```python
from build123d import *

# Parameters (mm, degrees)
F0_R     = 3.81
F1_DEPTH = 1.27


with BuildPart() as f1:
    # F0 (on Top) → F1 (new body)
    with BuildSketch(Plane.XY):
        with BuildLine():
            ThreePointArc((8.255, -3.299557), (8.729807, -1.680052), (8.89, 0))
            ThreePointArc((8.89, 0), (8.729807, 1.680052), (8.255, 3.299557))
            ThreePointArc((8.255, 3.299557), (7.698966, 4.445), (6.985, 5.499261))
            ThreePointArc((6.985, 5.499261), (4.445, 7.698966), (1.27, 8.798818))
            ThreePointArc((1.27, 8.798818), (0, 8.89), (-1.27, 8.798818))
            ThreePointArc((-1.27, 8.798818), (-4.445, 7.698966), (-6.985, 5.499261))
            ThreePointArc((-6.985, 5.499261), (-7.698966, 4.445), (-8.255, 3.299557))
            ThreePointArc((-8.255, 3.299557), (-8.89, 0), (-8.255, -3.299557))
            ThreePointArc((-8.255, -3.299557), (-7.698966, -4.445), (-6.985, -5.499261))
            ThreePointArc((-6.985, -5.499261), (-4.445, -7.698966), (-1.27, -8.798818))
            ThreePointArc((-1.27, -8.798818), (0, -8.89), (1.27, -8.798818))
            ThreePointArc((1.27, -8.798818), (4.445, -7.698966), (6.985, -5.499261))
            ThreePointArc((6.985, -5.499261), (7.698966, -4.445), (8.255, -3.299557))
        make_face()
        Circle(F0_R, mode=Mode.SUBTRACT)
        with BuildLine():
            ThreePointArc((-1.27, 8.798818), (0, 8.89), (1.27, 8.798818))
            Line((1.27, 8.798818), (1.27, 11.338818))
            Line((1.27, 11.338818), (-1.27, 11.338818))
            Line((-1.27, 11.338818), (-1.27, 8.798818))
        make_face()
        with BuildLine():
            ThreePointArc((6.985, 5.499261), (7.698966, 4.445), (8.255, 3.299557))
            Line((8.255, 3.299557), (10.454705, 4.569557))
            Line((10.454705, 4.569557), (9.184705, 6.769261))
            Line((9.184705, 6.769261), (6.985, 5.499261))
        make_face()
        with BuildLine():
            Line((10.454705, -4.569557), (8.255, -3.299557))
            ThreePointArc((8.255, -3.299557), (7.698966, -4.445), (6.985, -5.499261))
            Line((6.985, -5.499261), (9.184705, -6.769261))
            Line((9.184705, -6.769261), (10.454705, -4.569557))
        make_face()
        with BuildLine():
            Line((1.27, -11.338818), (1.27, -8.798818))
            ThreePointArc((1.27, -8.798818), (0, -8.89), (-1.27, -8.798818))
            Line((-1.27, -8.798818), (-1.27, -11.338818))
            Line((-1.27, -11.338818), (1.27, -11.338818))
        make_face()
        with BuildLine():
            Line((-9.184705, -6.769261), (-6.985, -5.499261))
            ThreePointArc((-6.985, -5.499261), (-7.698966, -4.445), (-8.255, -3.299557))
            Line((-8.255, -3.299557), (-10.454705, -4.569557))
            Line((-10.454705, -4.569557), (-9.184705, -6.769261))
        make_face()
        with BuildLine():
            ThreePointArc((-8.255, 3.299557), (-7.698966, 4.445), (-6.985, 5.499261))
            Line((-6.985, 5.499261), (-9.184705, 6.769261))
            Line((-9.184705, 6.769261), (-10.454705, 4.569557))
            Line((-10.454705, 4.569557), (-8.255, 3.299557))
        make_face()
    extrude(amount=F1_DEPTH)


solid = f1.part
```
The listing builds one solid part. Answer for the finished solid, in the listing's coordinates (mm). A direction names the side the tool comes from. Give positions to 0.01 mm unless a question says otherwise; leave off trailing zeros. Order: outer loops, then holes, each group sorted by start corner. A loop starts at its lowest first (then second) coordinate and runs counter-clockwise, first axis right, second up. Notation, with made-up numbers: (-23.75, 82) -> (-11.75, 82) arc R24 cw to (-11.75, 117) -> close; hole circle Ø8 at (31.25, 54). An arc over 180 degrees is marked (long way). Answer as a JSON object with one key per item and string values. Group by question number.
Item 1: The part is cut by section A-A on x = 0. Write down the section's boundary in (y, z).
Item 2: Consider L1, parallel to Y at x = 0, z = 0.6; L2, parallel to X at y = 6.5, z = 0.1; L3, parallel to X at y = -0.75, z = 0.5. Determine where each line is inside the solid, lowest interval first. Write a range as from..to.
Item 3: The part is cut by section D-D on y = 10.25. Write down the section's boundary in (x, z), and give its area (3 significant figures).
Item 4: Determine the mould class of faces 5 (the flat face through (9.37, -3.943, 0.626)), 6 (the flat face through (-9.8, 5.7, 0.6)), 7 (the flat face through (1.27, 10, 1)) for opening direction Y: pulls with the +Y half, pulls with the -Y half, needs draft (parallel to the pull), parting line crosses it, or undercut.
Item 5: A tool of negligible diameter and unlimited length cuts with its end or side. For faces 1 (the flat face through (1.27, -10, 1)), 2 (the cylindrical face through (-4.404, 7.723, 0.626)), 3 (the flat face through (-1.27, 10, 1)), 4 (the flat face through (-8.1, -6.143, 0.626)), from which of +Z, -Z, +X, -X, +Y, -Y can it reach the whole face along a straight path? Write none if from no direction.
Item 6: Flat-ended cylindrical pins translate along their axes: pin 1 (8 mm diameter, centred on x = -6, y = 7, fed in from +Z); pin 2 (0.6 mm diameter, centred on y = 10.5, z = 0.5, fed in from -X). Find the tip coordinate at first contact, or state that the pin passes through.
Item 7: The part is cut by section C-C on y = 2.25. Write down the section's boundary in (x, z), and give its area (3 significant figures).
Item 8: The part is cut by section B-B on z = 0.4. Write down the section's boundary in (x, y) (3 decimals), and give its area (3 significant figures).
Result set:
{
 "1": {"outline": "(-11.34, 0) -> (-3.81, 0) -> (-3.81, 1.27) -> (-11.34, 1.27) -> close; (3.81, 0) -> (11.34, 0) -> (11.34, 1.27) -> (3.81, 1.27) -> close"},
 "2": {"L1": "-11.34..-3.81, 3.81..11.34", "L2": "-9.34..-8.72, -6.06..6.06, 8.72..9.34", "L3": "-8.86..-3.74, 3.74..8.86"},
 "3": {"outline": "(-1.27, 0) -> (1.27, 0) -> (1.27, 1.27) -> (-1.27, 1.27) -> close", "area": "3.23 mm²"},
 "4": {"face 5": "undercut", "face 6": "pulls with the +Y half", "face 7": "needs draft"},
 "5": {"face 1": "+Z, -Z, +X, -Y", "face 2": "+Z, -Z, +Y", "face 3": "+Z, -Z, -X, +Y", "face 4": "+Z, -Z, -Y"},
 "6": {"pin 1": "z = 1.27", "pin 2": "x = -1.27"},
 "7": {"outline": "(-8.6, 0) -> (-3.07, 0) -> (-3.07, 1.27) -> (-8.6, 1.27) -> close; (3.07, 0) -> (8.6, 0) -> (8.6, 1.27) -> (3.07, 1.27) -> close", "area": "14.0 mm²"},
 "8": {"outline": "(-10.455, -4.57) -> (-9.185, -6.769) -> (-6.985, -5.499) arc R8.89 ccw to (-1.27, -8.799) -> (-1.27, -11.339) -> (1.27, -11.339) -> (1.27, -8.799) arc R8.89 ccw to (6.985, -5.499) -> (9.185, -6.769) -> (10.455, -4.57) -> (8.255, -3.3) arc R8.89 ccw to (8.89, 0) arc R8.89 ccw to (8.255, 3.3) -> (10.455, 4.57) -> (9.185, 6.769) -> (6.985, 5.499) arc R8.89 ccw to (1.27, 8.799) -> (1.27, 11.339) -> (-1.27, 11.339) -> (-1.27, 8.799) arc R8.89 ccw to (-6.985, 5.499) -> (-9.185, 6.769) -> (-10.455, 4.57) -> (-8.255, 3.3) arc R8.89 ccw to (-8.255, -3.3) -> close; hole circle Ø7.62 at (0, 0)", "area": "240 mm²"}
}
